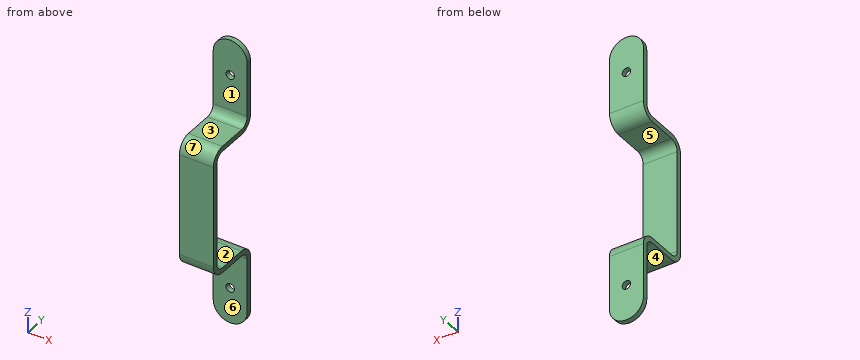
```python
from build123d import *

# Parameters (mm, degrees)
BASE_FLANGE1_DEPTH = 20
SKETCH6_R          = 2.5
CUT_EXTRUDE1_DEPTH = 10
FILLET1_R          = 10


# Sheet-metal steps are written as plain solids
with BuildPart() as part:
    # Sketch1 → Base-Flange1 (new body)
    with BuildSketch(Plane(origin=(0, 0, 0), x_dir=(0, 0, -1), z_dir=(1, 0, 0))):
        with BuildLine():
            Line((-85, 0), (-43, 0))
            ThreePointArc((-43, 0), (-37.343145751, -2.343145751), (-35, -8))
            Line((-35, -8), (-35, -25))
            ThreePointArc((-35, -25), (-33.535533906, -28.535533906), (-30, -30))
            Line((-30, -30), (30, -30))
            ThreePointArc((30, -30), (33.535533906, -28.535533906), (35, -25))
            Line((35, -25), (35, -8))
            ThreePointArc((35, -8), (37.343145751, -2.343145751), (43, 0))
            Line((43, 0), (85, 0))
            Line((85, 0), (85, -3))
            Line((85, -3), (43, -3))
            ThreePointArc((43, -3), (39.464466094, -4.464466094), (38, -8))
            Line((38, -8), (38, -25))
            ThreePointArc((38, -25), (35.656854249, -30.656854249), (30, -33))
            Line((30, -33), (-30, -33))
            ThreePointArc((-30, -33), (-35.656854249, -30.656854249), (-38, -25))
            Line((-38, -25), (-38, -8))
            ThreePointArc((-38, -8), (-39.464466094, -4.464466094), (-43, -3))
            Line((-43, -3), (-85, -3))
            Line((-85, -3), (-85, 0))
        make_face()
    extrude(amount=BASE_FLANGE1_DEPTH)

    # Sketch6 → Cut-Extrude1 (cut)
    with BuildSketch(Plane(origin=(0, 0, 0), x_dir=(1, 0, 0), z_dir=(0, 1, 0))):
        with Locations(Location((10, 64, 0), (0, 0, 270))):
            Circle(SKETCH6_R)
        with Locations(Location((10, -64, 0), (0, 0, 90))):
            Circle(SKETCH6_R)
    extrude(amount=-CUT_EXTRUDE1_DEPTH, mode=Mode.SUBTRACT)

    # Fillet1
    fillet1_edges = [part.edges().sort_by_distance(p)[0] for p in [
        (20, -1.5, -85),
        (0, -1.5, -85),
        (0, -1.5, 85),
        (20, -1.5, 85),
    ]]
    fillet(fillet1_edges, radius=FILLET1_R - 0.0001)  # a hair under: the kernel refuses the full size


solid = part.part
```
The listing builds one solid part. Answer for the finished solid, in the listing's coordinates (mm). Face numbers are marked on the shaded views. A direction names the side the tool comes from. Give positions to 0.01 mm unless a question says otherwise; leave off trailing zeros. Write each loop counter-clockwise with the first axis right and the second up, starting at its lowest first coordinate (ties: lowest second). Pieces come first, ordered by that corner, then holes. Notation, with made-up numbers: (-3.75, 28.25) - (11.25, 28.25) arc R9 ccw to (11.25, 40.25) - close; hole circle Ø6 at (-14.75, 2). An arc over 180 degrees is marked (long way). Use one line per item in the form item = value. Start each with the question number.
1) Find section A-A on z = -64. Determine the outline of the cut face in (x, y).
2) Flat-ended cylindrical pins translate along their axes: pin 1 Ø8.5 at (x, y) = (8, -18) entering from -Z; pin 2 Ø4 at (x, y) = (13, -8.5) entering from +Z; pin 3 Ø10 at (x, y) = (16.5, -6.5) entering from -Z. Find the tip coordinate at first contact, or state that the pin passes through.
3) Consider line 1 along Z through (x, y) = (6.75, -25); line 2 along X through (y, z) = (-1, 64); line 3 along Y through (x, z) = (15, 59.5). Determine where each line is inside the solid, lowest interval first. Write a range as from..to.
4) A tool of negligible diameter and unlimited length cuts with its end or side. For the marked faces 5, 6 and 7, from which of +Z, -Z, +X, -X, +Y, -Y can it reach the whole face along a straight path? Write none if from no direction.
5) Find section C-C on x = 4. Determine the outline of the cut face in (y, z).
6) Find section B-B on y = -15.5. Determine the outline of the cut face in (x, z).
7) Find section D-D on z = 21.5. Determine the outline of the cut face in (x, y), plus the area to 3 significant figures.
8) The mould has two halves that part along Z. Classify the marked faces 1, 2, 3 and 4: pulls with the +Z half, pulls with the -Z half, needs draft (parallel to the pull), parting line crosses it, or undercut.
Geometry results:
q1.outline = (0, -3) - (7.5, -3) - (7.5, 0) - (0, 0) - close; (12.5, -3) - (20, -3) - (20, 0) - (12.5, 0) - close
q2.pin_1 = -38
q2.pin_2 = 38.23
q2.pin_3 = -84.56
q3.line_1 = -38..-35, 35..38
q3.line_2 = 0..7.5, 12.5..20
q3.line_3 = -3..0
q4.face_5 = +X, -X, +Y
q4.face_6 = -Z, +X, -X, -Y
q4.face_7 = +Z, +X, -X, -Y
q5.outline = (-33, -30) arc R8 ccw to (-25, -38) - (-8, -38) arc R5 cw to (-3, -43) - (-3, -83) - (0, -83) - (0, -43) arc R8 ccw to (-8, -35) - (-25, -35) arc R5 cw to (-30, -30) - (-30, 30) arc R5 cw to (-25, 35) - (-8, 35) arc R8 ccw to (0, 43) - (0, 83) - (-3, 83) - (-3, 43) arc R5 cw to (-8, 38) - (-25, 38) arc R8 ccw to (-33, 30) - close
q6.outline = (0, -38) - (20, -38) - (20, -35) - (0, -35) - close; (0, 35) - (20, 35) - (20, 38) - (0, 38) - close
q7.outline = (0, -33) - (20, -33) - (20, -30) - (0, -30) - close
q7.area = 60.0 mm2
q8.face_1 = needs draft
q8.face_2 = undercut
q8.face_3 = pulls with the +Z half
q8.face_4 = pulls with the -Z half
